Source: CAD feature listing. Evaluate the final solid. Frame: model axes, mm. A direction names the side the tool comes from. Coordinates: 2 decimals unless noted, no trailing zeros. Loops run counter-clockwise (first coordinate to the right, second up) from the corner with the lowest first, then second, coordinate; pieces in that order, holes last.
from build123d import *

# Parameters (mm, degrees)
EXTRUDE_1_DEPTH     = 30
CUT_EXTRUDE_1_REACH = 522
SKETCH_2_R          = 12.5
CUT_EXTRUDE_2_REACH = 522
SKETCH_3_R          = 12.5
SKETCH_5_R          = 3
CUT_EXTRUDE_3_DEPTH = 5
SKETCH_6_R          = 3
CUT_EXTRUDE_5_DEPTH = 5
SKETCH_7_R          = 3
CUT_EXTRUDE_6_DEPTH = 5


with BuildPart() as part:
    # 草图1 → Extrude 1 (new body)
    with BuildSketch(Plane.XY):
        Polygon((-255, 204.5), (-255, -204.5), (255, -204.5), (255, 204.5), (260, 204.5), (260, -209.5), (-260, -209.5), (-260, 204.5), align=None)
    extrude(amount=EXTRUDE_1_DEPTH)

    # 草图2 → 切除-拉伸1 (cut, up to next)
    with BuildSketch(Plane.ZY.offset(260), mode=Mode.PRIVATE) as cut_extrude_1_sk1:
        with Locations((0, 40.5)):
            Circle(SKETCH_2_R)
    cut_extrude_1_tool1 = extrude(cut_extrude_1_sk1.sketch, amount=-CUT_EXTRUDE_1_REACH, mode=Mode.PRIVATE) & part.part
    add(cut_extrude_1_tool1.solids().sort_by_distance((-260, 40.5, 0))[0], mode=Mode.SUBTRACT)

    # 草图3 → 切除-拉伸2 (cut, up to next)
    with BuildSketch(Plane(origin=(260, 0, 0), x_dir=(0, 0, -1), z_dir=(1, 0, 0)), mode=Mode.PRIVATE) as cut_extrude_2_sk1:
        with Locations((0, 40.5)):
            Circle(SKETCH_3_R)
    cut_extrude_2_tool1 = extrude(cut_extrude_2_sk1.sketch, amount=-CUT_EXTRUDE_2_REACH, mode=Mode.PRIVATE) & part.part
    add(cut_extrude_2_tool1.solids().sort_by_distance((260, 40.5, 0))[0], mode=Mode.SUBTRACT)
    # 草图3 → 切除-拉伸2 (cut, up to next)
    with BuildSketch(Plane(origin=(260, 0, 0), x_dir=(0, 0, -1), z_dir=(1, 0, 0)), mode=Mode.PRIVATE) as cut_extrude_2_sk2:
        with Locations((0, -9.5)):
            Circle(SKETCH_3_R)
    cut_extrude_2_tool2 = extrude(cut_extrude_2_sk2.sketch, amount=-CUT_EXTRUDE_2_REACH, mode=Mode.PRIVATE) & part.part
    add(cut_extrude_2_tool2.solids().sort_by_distance((260, -9.5, 0))[0], mode=Mode.SUBTRACT)

    # 草图5 → 切除-拉伸3 (cut)
    with BuildSketch(Plane(origin=(260, 0, 0), x_dir=(0, 0, -1), z_dir=(1, 0, 0))):
        with Locations((0, -29.5)):
            Circle(SKETCH_5_R)
        with Locations((-17.320508076, 0.5)):
            Circle(SKETCH_5_R)
    extrude(amount=-CUT_EXTRUDE_3_DEPTH, mode=Mode.SUBTRACT)

    # 草图6 → 切除-拉伸5 (cut)
    with BuildSketch(Plane.ZY.offset(260)):
        with Locations((0, 60.5)):
            Circle(SKETCH_6_R)
        with Locations((17.320508076, 30.5)):
            Circle(SKETCH_6_R)
    extrude(amount=-CUT_EXTRUDE_5_DEPTH, mode=Mode.SUBTRACT)

    # 草图7 → 切除-拉伸6 (cut)
    with BuildSketch(Plane(origin=(260, 0, 0), x_dir=(0, 0, -1), z_dir=(1, 0, 0))):
        with Locations((0, 63.5)):
            Circle(SKETCH_7_R)
        with Locations((-19.918584287, 29)):
            Circle(SKETCH_7_R)
    extrude(amount=-CUT_EXTRUDE_6_DEPTH, mode=Mode.SUBTRACT)


solid = part.part
Q1. Access query for faces 4 (the flat face through (260, 0, 11)), 5 (the cylindrical face through (257.535, -9.225, 12.497)), 6 (the flat face through (-4, -204.5, 15)). Directions: +Z, -Z, +X, -X, +Y, -Y. A direction counts if a zero-diameter tool reaches every point of the face in a straight line with its end or side. Return the directions, or none.
Q2. Contact query for flat-ended pins moving along their axis: pin 1 Ø5 at (y, z) = (0.5, 17.32) entering from +X; pin 2 Ø1.5 at (x, z) = (5.5, 21) entering from +Y; pin 3 Ø9.5 at (y, z) = (30.5, 17.32) entering from -X. Output: stop coordinate, or through.
Q3. Section B-B, the plane y = -84. Return the cut outline in (x, z), plus the area to 3 significant figures.
Q4. Section C-C, the plane x = 48. Return the cut outline in (y, z), plus the area to 3 significant figures.
Q5. Draft query along X for faces 1 (the cylindrical face through (-257.535, 40.225, 12.497)), 2 (the flat face through (255, -3, 15)), 3 (the flat face through (-260, -5, 15)). Return one class per face: +X half, -X half, draft (parallel to the pull), parting line (faces both ways), or undercut.
Q6. Section A-A, the plane y = -9.5. Return the cut outline in (x, z).
Q7. Line query: line 1 along X through (y, z) = (103, 20.5); line 2 along Y through (x, z) = (-108, 15); line 3 along X through (y, z) = (-10.5, 12). Output: solid intervals per line, ascending.
Derived:
1. face 4: +Z, -Z, +X, +Y, -Y
1. face 5: -Z, +X
1. face 6: +Z, -Z, +Y
2. pin 1: stops at x = -255
2. pin 2: stops at y = -204.5
2. pin 3: stops at x = -260
3. outline: (-260, 0) - (-255, 0) - (-255, 30) - (-260, 30) - close; (255, 0) - (260, 0) - (260, 30) - (255, 30) - close
3. area: 300 mm2
4. outline: (-209.5, 0) - (-204.5, 0) - (-204.5, 30) - (-209.5, 30) - close
4. area: 150 mm2
5. face 1: draft
5. face 2: undercut
5. face 3: -X half
6. outline: (-260, 0) - (-255, 0) - (-255, 30) - (-260, 30) - close; (255, 12.5) - (260, 12.5) - (260, 30) - (255, 30) - close
7. line 1: x = -260 to -255, 255 to 260
7. line 2: y = -209.5 to -204.5
7. line 3: x = -260 to -255
